Build history of the part. All positions in model axes, mm. Round coordinates to 2 decimals unless told otherwise and drop trailing zeros. Write each loop counter-clockwise with the first axis right and the second up, starting at its lowest first coordinate (ties: lowest second). Pieces come first, ordered by that corner, then holes.
Autodesk Inventor part; units mm, degrees
ref_plane "YZ Plane" through (0, 0, 0) normal (1, 0, 0) x (0, 1, 0)
ref_plane "XZ Plane" through (0, 0, 0) normal (0, 1, 0) x (-1, 0, 0)
ref_plane "XY Plane" through (0, 0, 0) normal (0, 0, 1) x (1, 0, 0)
sketch "Sketch1" plane through (0, 0, 0) normal (0, 0, 1) x (1, 0, 0)
  line L0 (5, 2.8868) -> (5, -2.8868)
  line L1 (5, 2.8868) -> (0, 5.7735)
  line L2 (-5, 2.8868) -> (0, 5.7735)
  line L3 (0, -5.7735) -> (5, -2.8868)
  line L4 (-5, 2.8868) -> (-5, -2.8868)
  line L5 (-5, -2.8868) -> (0, -5.7735)
  point P0 (0, 0)
  point P1 (0, 0)
  point P2 (0, 0)
  point P3 (0, 0)
  point P4 (0, 0)
  dimension "d0" = 120
  dimension "d1" = 120
  dimension "d2" = 120
  dimension "d3" = 120
  dimension "d4" = 120
  dimension "d5" = 120
  dimension "d6" = 10
  dimension "d7" = 5
extrude "Extrusion1" add sketch "Sketch1" along normal blind 4
sketch "Sketch2" plane through (0, 0, 4) normal (0, 0, 1) x (1, 0, 0)
  point P0 (0, 0)
  point P1 (0, 0)
hole "Hole1" at (0, 0, 4) direction (0, 0, -1) diameter 4.134 end through all
properties part number "M5-nut-4mm" material "Steel, Mild"
1) Slice it at A-A (y = 0). Write the cut outline in (x, z), plus the area to 3 significant figures.
Results:
outline: (-5, 0) - (-2.07, 0) - (-2.07, 4) - (-5, 4) - close; (2.07, 0) - (5, 0) - (5, 4) - (2.07, 4) - close
area: 23.5 mm2
2) Pin check, flat tip, straight feed: pin 1 Ø1 at (x, z) = (-2, 2.5) entering from -Y. Stop position of the tip, or through.
Results:
pin 1: stops at y = -4.91
3) Slice it at D-D (y = -3.25). Write the cut outline in (x, z).
Results:
outline: (-4.37, 0) - (4.37, 0) - (4.37, 4) - (-4.37, 4) - close
4) Wall check: L1, parallel to X at y = 0, z = 2.7; L2, parallel to Y at x = -1.75, z = 3.65; L3, parallel to X at y = -0.5, z = 2.9. Give the ranges that are in metal, low to high.
Results:
L1: x = -5 to -2.07, 2.07 to 5
L2: y = -4.76 to -1.1, 1.1 to 4.76
L3: x = -5 to -2.01, 2.01 to 5
5) Slice it at B-B (z = 1.85). Write the cut outline in (x, y).
Results:
outline: (-5, -2.89) - (0, -5.77) - (5, -2.89) - (5, 2.89) - (0, 5.77) - (-5, 2.89) - close; hole circle Ø4.13 at (0, 0)
6) Mould opens along Y. For faces 1 (the cylindrical face through (1.26, 1.64, 1.97)), 2 (the flat face through (-5, 0, 2)), 3 (the flat face through (-2.535, 4.31, 1.972)) say: released by +Y, released by -Y, zero draft, split by the parting line, or undercut.
Results:
face 1: undercut
face 2: zero draft
face 3: released by +Y
7) Slice it at C-C (x = 3). Write the cut outline in (y, z), plus the area to 3 significant figures.
Results:
outline: (-4.04, 0) - (4.04, 0) - (4.04, 4) - (-4.04, 4) - close
area: 32.3 mm2
